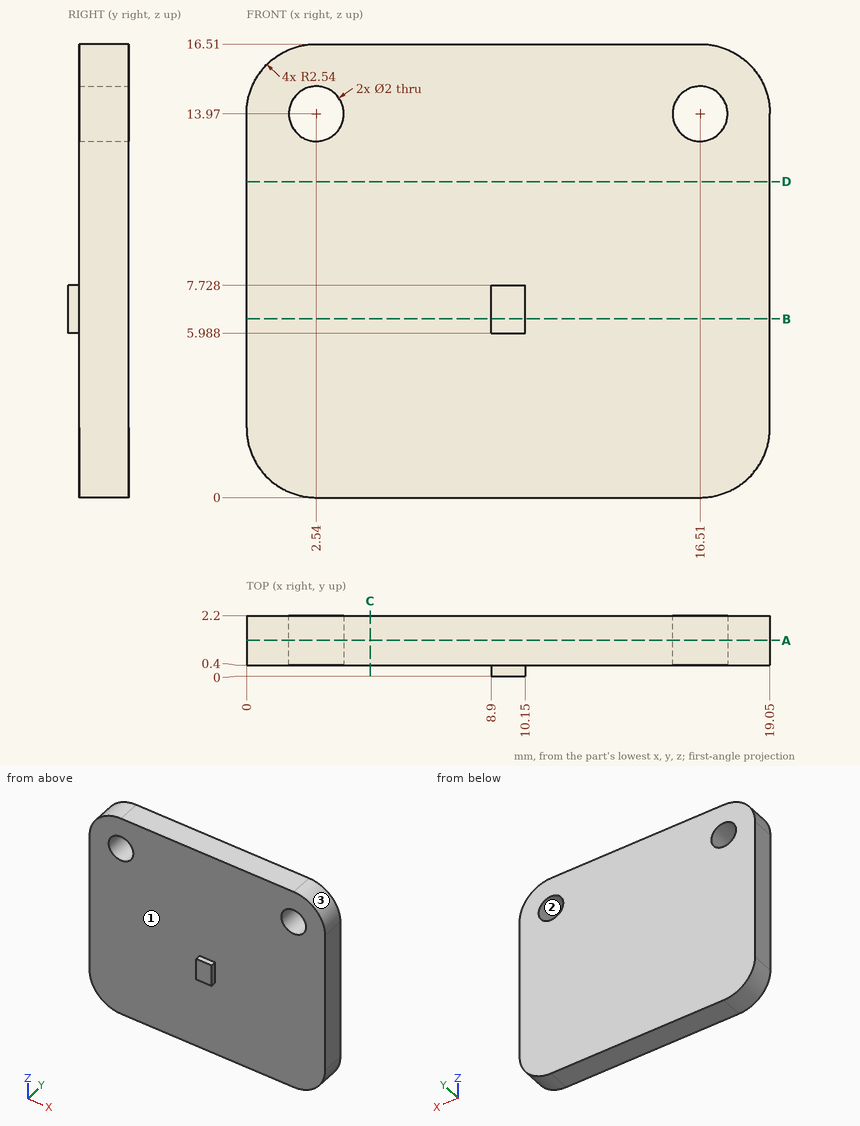
Design review of the part shown in the three views and the two pictorial views. Dimensions are in mm from the part's minimum x, y and z. Give positions to 0.01 mm unless a question says otherwise; leave off trailing zeros. Loops run counter-clockwise (first coordinate to the right, second up) from the corner with the lowest first, then second, coordinate; pieces in that order, holes last. Notation, with made-up numbers: (8.5, 30.5) -> (62.5, 30.5) arc R26 ccw to (62.5, 61.5) -> close; hole circle Ø7 at (84, -16). An arc over 180 degrees is marked (long way). Answer as a JSON object with one key per item and string values. Group by question number.
Q1. Take a section at A-A (y = 1.3). Write out the cut boundary in (x, z), plus the area to 3 significant figures.
Q2. Insertion check: pin 1 (2.5 mm diameter, centred on x = 2.54, z = 13.97, fed in from -Y). The pin has a flat end and moves straight along its axis. Give the tip position at first contact, or say it passes through.
Q3. Take a section at C-C (x = 4.5). Write out the cut boundary in (y, z).
Q4. Draft analysis for pull direction X (two halves, no side actions). For the marked faces 1, 2 and 3, state which applies: pulls with the +X half, pulls with the -X half, needs draft (parallel to the pull), parting line crosses it, or undercut.
Q5. Wall thickness on line 1 along Y through (x, z) = (6.5, 11); line 2 along Z through (x, y) = (9.75, 0.2); line 3 along Z through (x, y) = (17.25, 0.5): over which ranges is each line inside the solid? List them lowest first.
Q6. Take a section at D-D (z = 11.5). Write out the cut boundary in (x, y), plus the area to 3 significant figures.
Q7. Take a section at B-B (z = 6.5). Write out the cut boundary in (x, y), plus the area to 3 significant figures.
Answer below:
{
 "1": {"outline": "(0, 2.54) arc R2.54 ccw to (2.54, 0) -> (16.51, 0) arc R2.54 ccw to (19.05, 2.54) -> (19.05, 13.97) arc R2.54 ccw to (16.51, 16.51) -> (2.54, 16.51) arc R2.54 ccw to (0, 13.97) -> close; hole circle Ø2 at (2.54, 13.97); hole circle Ø2 at (16.51, 13.97)", "area": "303 mm2"},
 "2": {"pin 1": "stops at y = 0.4"},
 "3": {"outline": "(0.4, 0) -> (2.2, 0) -> (2.2, 16.51) -> (0.4, 16.51) -> close"},
 "4": {"face 1": "needs draft", "face 2": "undercut", "face 3": "pulls with the +X half"},
 "5": {"line 1": "y = 0.4 to 2.2", "line 2": "z = 5.99 to 7.73", "line 3": "z = 0.11 to 13.3, 14.64 to 16.4"},
 "6": {"outline": "(0, 0.4) -> (19.05, 0.4) -> (19.05, 2.2) -> (0, 2.2) -> close", "area": "34.3 mm2"},
 "7": {"outline": "(0, 0.4) -> (8.9, 0.4) -> (8.9, 0) -> (10.15, 0) -> (10.15, 0.4) -> (19.05, 0.4) -> (19.05, 2.2) -> (0, 2.2) -> close", "area": "34.8 mm2"}
}
